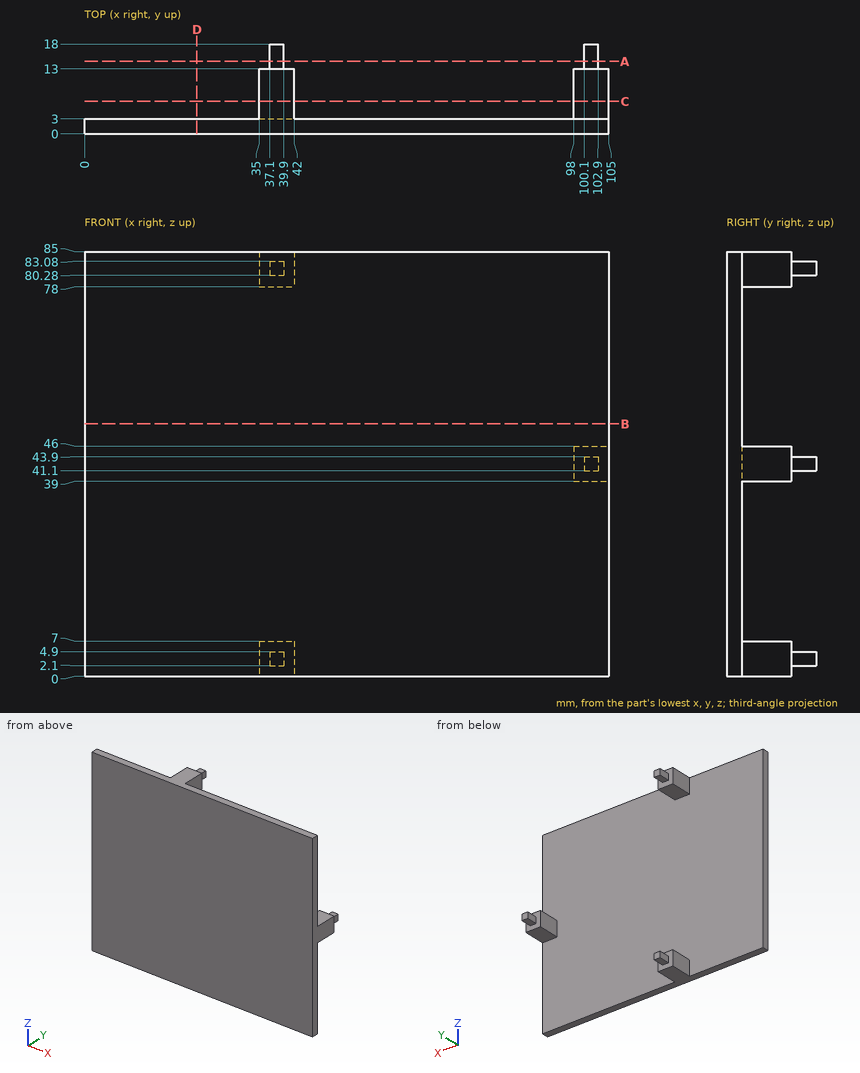
Drawing for the job (mm, zero at the part's lowest x, y, z). Give positions to 0.01 mm unless a question says otherwise; leave off trailing zeros. Loops run counter-clockwise (first coordinate to the right, second up) from the corner with the lowest first, then second, coordinate; pieces in that order, holes last.
Item 1: Slice it at D-D (x = 22.5). Write the cut outline in (y, z), plus the area to 3 significant figures.
Check values:
outline: (0, 0) - (3, 0) - (3, 85) - (0, 85) - close
area: 255 mm2
Item 2: Slice it at C-C (y = 6.5). Write the cut outline in (x, z).
Check values:
outline: (35, 0) - (42, 0) - (42, 7) - (35, 7) - close; (35, 78) - (42, 78) - (42, 85) - (35, 85) - close; (98, 39) - (105, 39) - (105, 46) - (98, 46) - close
Item 3: Drill centre lines: line 1 along X through (y, z) = (14.25, 4); line 2 along Y through (x, z) = (38, 68.5); line 3 along X through (y, z) = (6, 44). Where is each one in solid material? Low to high.
Check values:
line 1: x = 37.1 to 39.9
line 2: y = 0 to 3
line 3: x = 98 to 105
Item 4: Slice it at B-B (z = 50.5). Write the cut outline in (x, y).
Check values:
outline: (0, 0) - (105, 0) - (105, 3) - (0, 3) - close
Item 5: Slice it at A-A (y = 14.5). Write the cut outline in (x, z), plus the area to 3 significant figures.
Check values:
outline: (37.1, 2.1) - (39.9, 2.1) - (39.9, 4.9) - (37.1, 4.9) - close; (37.1, 80.28) - (39.9, 80.28) - (39.9, 83.08) - (37.1, 83.08) - close; (100.1, 41.1) - (102.9, 41.1) - (102.9, 43.9) - (100.1, 43.9) - close
area: 23.5 mm2
Item 6: Drop flat-ended pins along their axis: P1, Ø1.4, axis at x = 38.5, y = 15.5, coming from the -Z side; P2, Ø2, axis at y = 9, z = 5, coming from the +X side; P3, Ø0.8, axis at y = 14.5, z = 42.5, coming from the +X side. Give the stop position or say it passes through.
Check values:
P1: stops at z = 2.1
P2: stops at x = 42
P3: stops at x = 102.9
